Autodesk Fusion 360 part; units mm, degrees
sketch "Sketch1" plane through (0, 0, 0) normal (0, 0, 1) x (1, 0, 0)
  circle A0 centre (0, 0) radius 90
  circle A1 centre (0, 65) radius 10
  circle A2 centre (0, -65) radius 10
  circle A3 centre (0, 0) radius 25
  circle A4 centre (0, 0) radius 35
  circle A5 centre (0, 65) radius 20
  circle A6 centre (0, -65) radius 20
  line L0 (-10, 30) -> (10, 30)
  line L1 (10, 30) -> (10, 50)
  line L2 (10, 50) -> (-10, 50)
  line L3 (-10, 50) -> (-10, 30)
  line L4 (-10, -30) -> (10, -30)
  line L5 (10, -30) -> (10, -50)
  line L6 (10, -50) -> (-10, -50)
  line L7 (-10, -50) -> (-10, -30)
  dimension "d1" = 50
sketch "Sketch2" plane through (0, 0, 0) normal (0, 0, 1) x (1, 0, 0)
sketch "Sketch3" plane through (0, 0, 0) normal (0, 0, 1) x (1, 0, 0)
  circle A0 centre (0, 0) radius 30
sketch "Sketch4" plane through (0, 0, 0) normal (0, 0, 1) x (1, 0, 0)
sketch "Sketch5" plane through (0, 0, 0) normal (0, 1, 0) x (1, 0, 0)
sketch "Sketch6" plane through (0, 0, 0) normal (0, 0, 1) x (1, 0, 0)
  circle A0 centre (0, 65) radius 5.25
  circle A1 centre (0, 65) radius 10
  dimension "d6" = 10.5
sketch "Sketch7" plane through (0, 0, 0) normal (0, 0, 1) x (1, 0, 0)
  circle A0 centre (0, -65) radius 5.25
  circle A1 centre (0, -65) radius 10
  dimension "d9" = 10.5
sketch "Sketch8" plane through (0, 0, 0) normal (0, 0, 1) x (1, 0, 0)
  circle A0 centre (0, 0) radius 40
  circle A1 centre (0, 0) radius 30
  circle A2 centre (0, 0) radius 30
sketch "Sketch9" plane through (0, 0, 0) normal (0, 0, 1) x (1, 0, 0)
sketch "Sketch10" plane through (0, 0, 0) normal (0, 0, 1) x (1, 0, 0)
sketch "Sketch11" plane through (0, 0, 0) normal (0, 0, 1) x (1, 0, 0)
sketch "Sketch12" plane through (0, 0, 0) normal (0, 0, 1) x (1, 0, 0)
  circle A0 centre (0, 65) radius 15
  circle A1 centre (0, 65) radius 20
sketch "Sketch13" plane through (0, 0, 0) normal (0, 0, 1) x (1, 0, 0)
  circle A0 centre (0, -65) radius 15
  circle A1 centre (0, -65) radius 20
extrude "Extrude7" cut sketch "Sketch13" along normal blind 22
sketch "Sketch14" plane through (0, 0, 0) normal (0, 0, 1) x (1, 0, 0)
  line L0 (-10, -35) -> (10, -35)
  line L1 (10, -35) -> (10, -59)
  line L2 (10, -59) -> (-10, -59)
  line L3 (-10, -59) -> (-10, -35)
  line L4 (-10, 35) -> (10, 35)
  line L5 (10, 35) -> (10, 58)
  line L6 (10, 58) -> (-10, 58)
  line L7 (-10, 58) -> (-10, 35)
sketch "Sketch15" plane through (0, 0, 0) normal (0, 0, 1) x (1, 0, 0)
sketch "Sketch16" plane through (0, 0, 0) normal (0, 0, 1) x (1, 0, 0)
sketch "Sketch17" plane through (0, 0, 0) normal (0, 0, 1) x (1, 0, 0)
sketch "Sketch18" plane through (0, 0, 0) normal (0, 0, 1) x (1, 0, 0)
  line L0 (0, -60) -> (0, 60)
  circle A0 centre (0, 0) radius 40
  circle A1 centre (0, 0) radius 30
  circle A2 centre (0, 70) radius 5
  circle A3 centre (0, -70) radius 5
  circle A4 centre (0, 70) radius 15
  circle A5 centre (0, -70) radius 15
sketch "Sketch19" plane through (0, 0, 0) normal (0, 0, 1) x (1, 0, 0)
extrude "Extrude9" add sketch "Sketch18" along normal blind 5 separate body contours A4 | L0 A0 A1 | L0 A0 A1 | A5 makes body 1 at (11.5922, -69.0064, 5) makes body 2 at (36.4061, -3.4777, 5) makes body 3 at (11.6108, 69.2548, 0)
sketch "Sketch20" plane through (0, 0, 0) normal (0, 0, 1) x (1, 0, 0)
  line L0 (-7, -37) -> (8, -37)
  line L1 (8, -37) -> (8, -59)
  line L2 (8, -59) -> (-7, -59)
  line L3 (-7, -59) -> (-7, -37)
  line L4 (8, -37) -> (-8, -37)
  line L5 (-8, -37) -> (-8, -59)
  line L6 (-8, -59) -> (8, -59)
  line L7 (8, -59) -> (8, -37)
  line L8 (-8, 37) -> (7, 37)
  line L9 (7, 37) -> (7, 61)
  line L10 (7, 61) -> (-8, 61)
  line L11 (-8, 61) -> (-8, 37)
  line L12 (-5, 38) -> (5, 38)
  line L13 (5, 38) -> (5, 59)
  line L14 (5, 59) -> (-5, 59)
  line L15 (-5, 59) -> (-5, 38)
  line L16 (5, -35) -> (-5, -35)
  line L17 (-5, -35) -> (-5, -59)
  line L18 (-5, -59) -> (5, -59)
  line L19 (5, -59) -> (5, -35)
extrude "Extrude10" add sketch "Sketch20" along normal blind 5 contours L0 L2 L4 L6 L17 L18 L19 | L12 L13 L14 L15 bodies 1 2 3
Check sheet for the modelled part. Datum: model origin and axes. Units: mm. A direction names the side the tool comes from. Coordinates: 2 decimals unless noted, no trailing zeros. Order: outer loops, then holes, each group sorted by start corner. A loop starts at its lowest first (then second) coordinate and runs counter-clockwise, first axis right, second up. Notation, with made-up numbers: (-23.5, 15.5) -> (10.5, 15.5) arc R21 ccw to (10.5, 26.5) -> close; hole circle Ø6 at (52.5, -33). An arc over 180 degrees is marked (long way). Write item = value, one per line. Start each with the question number.
1) Cross-section at D-D (y = -72.5). Enter the section's corners in (x, z).
2) Material ranges on L1, parallel to Y at x = 0, z = 1.1; L2, parallel to X at y = 0, z = 3.55; L3, parallel to Y at x = 12.5, z = 0.35, recorded low to high.
3) Go/stop test with flat-tipped pins: P1, Ø1.5, axis at y = 48, z = 1.5, coming from the +X side; P2, Ø8, axis at x = 0, y = -70, coming from the -Z side; P3, Ø1, axis at x = 14, z = 4.5, coming from the +Y side; P4, Ø1.5, axis at y = -29.5, z = 2, coming from the -X side. Record where each tip stops, or that it passes through.
4) Cross-section at C-C (x = 0). Enter the section's corners in (y, z), then the cut area to 3 significant figures.
5) Mould release check, pull along X, two halves, no side actions. Record for faces 4 (the flat face through (-5, 48, 2)), 5 (the cylindrical face through (0.59, -84.99, 2.46)), 6 (the cylindrical face through (3, 66, 2)), 7 (the cylindrical face through (-29.97, -1.32, 2.46)): +X half, -X half, draft (parallel to the pull), parting line (faces both ways), or undercut.
6) Access from +Z, -Z, +X, -X, +Y, -Y to the whole of each face (thin tool, end or side, straight path). Record for faces 1 (the cylindrical face through (-1.08, -65.12, 2.46)), 2 (the flat face through (-5, -48, 2)), 3 (the flat face through (5, -48, 2)).
7) Cross-section at A-A (y = 0). Enter the section's corners in (x, z).
8) Cross-section at B-B (z = 2.9). Enter the section's corners in (x, y), then the cut area to 3 significant figures.
Ans:
q1.outline = (-14.79, 0) -> (-4.33, 0) -> (-4.33, 5) -> (-14.79, 5) -> close; (4.33, 0) -> (14.79, 0) -> (14.79, 5) -> (4.33, 5) -> close
q2.L1 = -85 to -75, -65 to -30, 30 to 65, 75 to 85
q2.L2 = -40 to -30, 30 to 40
q2.L3 = -78.29 to -61.71, -38 to -27.27, 27.27 to 38, 61.71 to 78.29
q3.P1 = 5
q3.P2 = through
q3.P3 = 76.54
q3.P4 = -27.81
q4.outline = (-85, 0) -> (-75, 0) -> (-75, 5) -> (-85, 5) -> close; (-65, 0) -> (-30, 0) -> (-30, 5) -> (-65, 5) -> close; (30, 0) -> (65, 0) -> (65, 5) -> (30, 5) -> close; (75, 0) -> (85, 0) -> (85, 5) -> (75, 5) -> close
q4.area = 450 mm²
q5.face_4 = -X half
q5.face_5 = parting line
q5.face_6 = undercut
q5.face_7 = undercut
q6.face_1 = +Z, -Z
q6.face_2 = +Z, -Z, -X
q6.face_3 = +Z, -Z, +X
q7.outline = (-40, 0) -> (-30, 0) -> (-30, 5) -> (-40, 5) -> close; (30, 0) -> (40, 0) -> (40, 5) -> (30, 5) -> close
q8.outline = (-5, -55.86) arc R15 ccw (long way) to (5, -55.86) -> (5, -39.69) arc R40 ccw to (5, 39.69) -> (5, 55.86) arc R15 ccw (long way) to (-5, 55.86) -> (-5, 39.69) arc R40 ccw to (-5, -39.69) -> close; hole circle Ø60 at (0, 0); hole circle Ø10 at (0, -70); hole circle Ø10 at (0, 70)
q8.area = 3,760 mm²
